Model file for the job. Use its own axes, mm. Coordinates: 2 decimals unless noted, no trailing zeros. Order: outer loops, then holes, each group sorted by start corner. A loop starts at its lowest first (then second) coordinate and runs counter-clockwise, first axis right, second up.
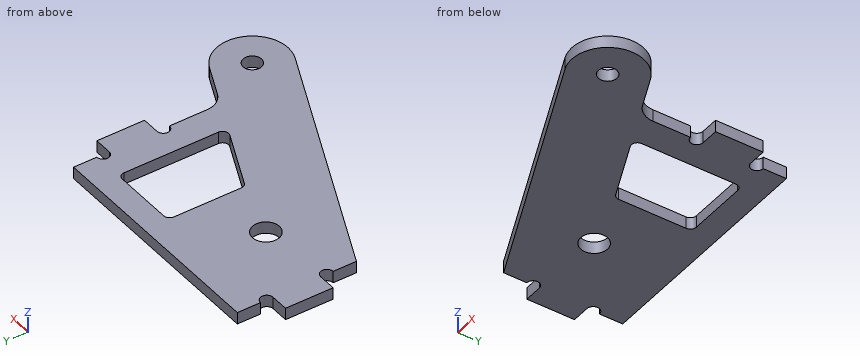
Autodesk Inventor part; units mm, degrees
ref_plane "YZ Plane" through (0, 0, 0) normal (1, 0, 0) x (0, 1, 0)
ref_plane "XZ Plane" through (0, 0, 0) normal (0, 1, 0) x (-1, 0, 0)
ref_plane "XY Plane" through (0, 0, 0) normal (0, 0, 1) x (1, 0, 0)
sketch "スケッチ1" plane through (0, 0, 0) normal (0, 0, 1) x (1, 0, 0)
  line L0 (-19.75, 25.75) -> (19.75, 25.75) construction
  line L1 (19.75, 25.75) -> (19.75, -25.75) construction
  line L2 (19.75, -25.75) -> (-19.75, -25.75) construction
  line L3 (-19.75, -25.75) -> (-19.75, 25.75) construction
  line L4 (-19.75, 25.75) -> (19.75, -25.75) construction
  line L5 (19.75, 25.75) -> (-19.75, -25.75) construction
  circle A0 centre (24.75, -24.25) radius 1.55
  circle A1 centre (-7.25, -4.25) radius 2.25
  line L6 (0, 25.75) -> (0, -25.75) construction
  line L7 (-19.75, 3.25) -> (-22.75, 3.25)
  line L8 (-22.75, 3.25) -> (-22.75, -4.75)
  arc A2 (-19.75, 3.25) -> (-19.75, 5.35) centre (-19.75, 4.3) ccw
  line L9 (-22.75, -0.75) -> (-19.75, -0.75) construction
  line L10 (-19.75, -4.75) -> (-22.75, -4.75)
  arc A3 (-19.75, -6.85) -> (-19.75, -4.75) centre (-19.75, -5.8) ccw
  line L11 (-19.75, 5.35) -> (-19.75, 9.25)
  line L12 (-19.75, 9.25) -> (19.75, 9.25)
  arc A4 (19.75, 5.35) -> (19.75, 3.25) centre (19.75, 4.3) ccw
  arc A5 (19.75, -4.75) -> (19.75, -6.85) centre (19.75, -5.8) ccw
  line L13 (19.75, 5.35) -> (19.75, 9.25)
  arc A6 (22.2819, -29.7189) -> (27.2181, -18.7811) centre (24.75, -24.25) ccw
  line L14 (-19.75, -6.85) -> (-19.75, -10.75)
  line L15 (-19.75, -10.75) -> (22.2819, -29.7189)
  line L16 (19.75, -6.85) -> (19.75, -15.4108)
  line L17 (19.75, -15.4108) -> (27.2181, -18.7811)
  circle A7 centre (-7.25, -4.25) radius 6 construction
  circle A8 centre (24.75, -24.25) radius 6 construction
  line L18 (2.75, 5.25) -> (14.75, 5.25)
  line L19 (14.75, 5.25) -> (14.75, -13.1543)
  line L20 (14.75, -13.1543) -> (2.75, -7.7388)
  line L21 (2.75, -7.7388) -> (2.75, 5.25)
  line L22 (19.75, 3.25) -> (22.75, 3.25)
  line L23 (22.75, 3.25) -> (22.75, -4.75)
  line L24 (22.75, -4.75) -> (19.75, -4.75)
  point P0 (0, 0)
  dimension "d0" = 39.5
  dimension "d1" = 51.5
  dimension "d2" = 3.1
  dimension "d3" = 4.5
  dimension "d4" = 32
  dimension "d5" = 20
  dimension "d6" = 3
  dimension "d7" = 1.05
  dimension "d8" = 8
  dimension "d9" = 26.5
  dimension "d11" = 30
  dimension "d12" = 12.5
  dimension "d13" = 6
  dimension "d14" = 12
  dimension "d19" = 12
  dimension "d20" = 12
  dimension "d21" = 4
  dimension "d22" = 5
  dimension "d24" = 4
  dimension "d26" = 3
extrude "押し出し1" add sketch "スケッチ1" along normal blind 2
fillet "フィレット1" radius 3.5 1 edges at (19.75, -15.4108, 1)
fillet "フィレット2" radius 1 4 edges at (2.75, 5.25, 1) (14.75, 5.25, 1) (2.75, -7.7388, 1) (14.75, -13.1543, 1)
equation "\"d24\" = d21"
properties part number "Leg_joint_pitch_frame" material "アルミニウム 2014-T4"
Q1. Drop flat-ended pins along their axis: P1, Ø0.6, axis at x = 10, z = 1.5, coming from the -Y side; P2, Ø1, axis at y = 0, z = 1, coming from the +X side; P3, Ø1, axis at y = 8, z = 1, coming from the +X side. Give the stop position or say it passes through.
Established:
P1: stops at y = -24.31
P2: stops at x = 22.75
P3: stops at x = 19.75
Q2. Cut at A-A, the plane z = 0.65. Count the separate pieces of the cut face and the enclosed holes in it, plus the area to 3 significant figures.
Established:
separate pieces: 1
enclosed holes: 3
area: 1,100 mm2
Q3. Cut at B-B, the plane y = 1. List the corners of the cut face in (x, z), plus the area to 3 significant figures.
Established:
outline: (-22.75, 0) - (2.75, 0) - (2.75, 2) - (-22.75, 2) - close; (14.75, 0) - (22.75, 0) - (22.75, 2) - (14.75, 2) - close
area: 67.0 mm2
Q4. Cut at D-D, the plane y = -5.5. List the corners of the cut face in (x, z).
Established:
outline: (-18.74, 0) - (-9.12, 0) - (-9.12, 2) - (-18.74, 2) - close; (-5.38, 0) - (2.75, 0) - (2.75, 2) - (-5.38, 2) - close; (14.75, 0) - (18.74, 0) - (18.74, 2) - (14.75, 2) - close
Q5. Probe line 1 (X direction, y = -2.5, z = 1.45); line 2 (X direction, y = 3, z = 0.5); line 3 (Y direction, x = -8.5, z = 0.85). List the from-to ranges inside material, lowest first.
Established:
line 1: x = -22.75 to -8.66, -5.84 to 2.75, 14.75 to 22.75
line 2: x = -22.75 to 2.75, 14.75 to 22.75
line 3: y = -15.83 to -6.12, -2.38 to 9.25
Q6. Cut at C-C, the plane x = -7.25. List the corners of the cut face in (y, z).
Established:
outline: (-16.39, 0) - (-6.5, 0) - (-6.5, 2) - (-16.39, 2) - close; (-2, 0) - (9.25, 0) - (9.25, 2) - (-2, 2) - close
